Geometry: see drawing. Coordinates: mm, zero at the bounding-box minimum. A direction names the side the tool comes from. Give positions to 0.01 mm unless a question says otherwise; leave off trailing zeros. Loops run counter-clockwise (first coordinate to the right, second up) from the corner with the lowest first, then second, coordinate; pieces in that order, holes last. Notation, with made-up numbers: (7.5, 39) -> (36.5, 39) arc R23 ccw to (36.5, 48) -> close; hole circle Ø6 at (37, 70.5). An arc over 180 degrees is marked (long way). Return JSON: item names as keys, results as strings. Group by question number.
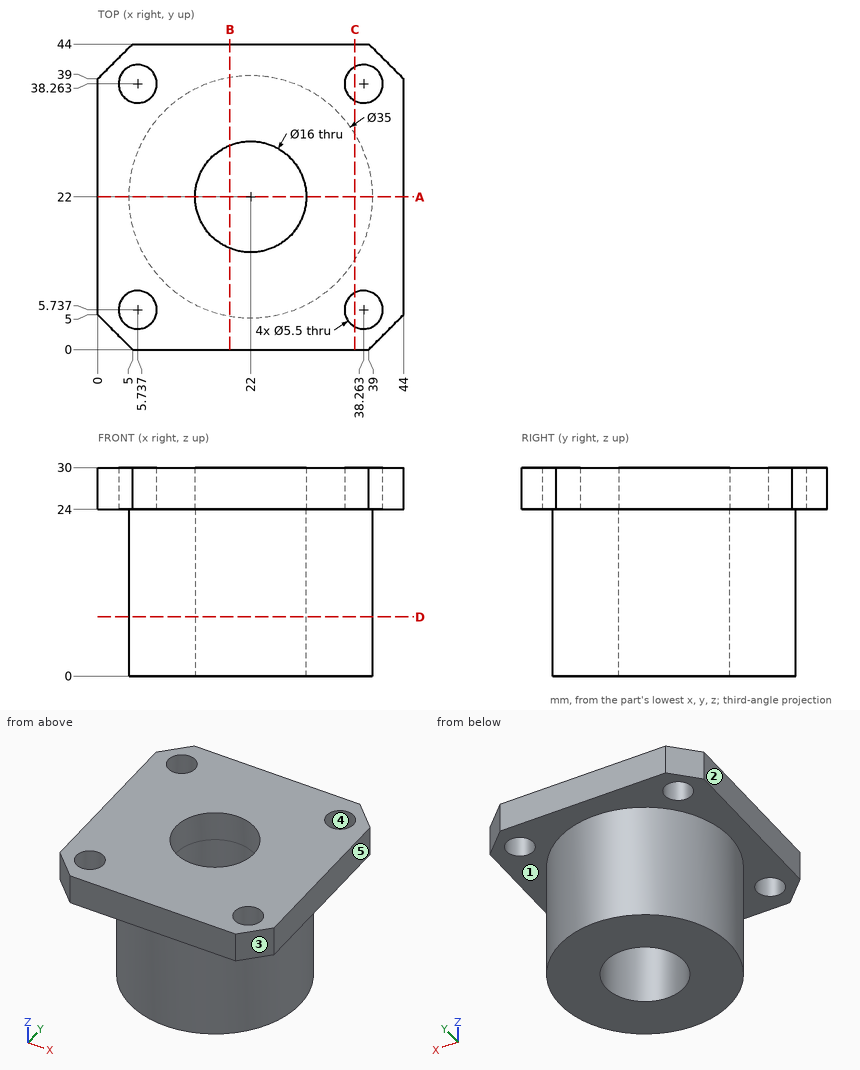
1) Mould query, pull axis Y, two halves, no side actions, for the marked faces 3, 4 and 5. Classes: released by +Y, released by -Y, zero draft, split by the parting line, or undercut.
2) Cut plane D-D on z = 8.5. Return loops of the section in (x, y), then the cut area to 3 significant figures.
3) Cut plane B-B on x = 19. Return loops of the section in (y, z).
4) Cut plane A-A on y = 22. Return loops of the section in (x, z), then the cut area to 3 significant figures.
5) Contact query for flat-ended pins moving along their axis: P1, Ø3, axis at x = 19.5, y = 7, coming from the -Z side; P2, Ø1.5, axis at y = 24, z = 19, coming from the -X side (1 decimal); P3, Ø7, axis at x = 5.74, y = 38.26, coming from the -Z side; P4, Ø4.5, axis at x = 5.74, y = 5.74, coming from the +Z side. Output: stop coordinate, or through.
6) Reachability of the marked faces 1 and 2 from +Z, -Z, +X, -X, +Y, -Y: full face, straight path, thin tool, end or side. Return the list, or none.
7) Cut plane C-C on x = 37. Return loops of the section in (y, z).
8) Material intervals for line 1 (Y direction, x = 22, z = 8.25); line 2 (Y direction, x = 22, z = 26); line 3 (Z direction, x = 37.5, y = 11.5), sorted ascending.
Calculated:
{
 "1": {"face 3": "released by -Y", "face 4": "undercut", "face 5": "zero draft"},
 "2": {"outline": "circle Ø35 at (22, 22); hole circle Ø16 at (22, 22)", "area": "761 mm2"},
 "3": {"outline": "(0, 24) -> (4.76, 24) -> (4.76, 0) -> (14.58, 0) -> (14.58, 30) -> (0, 30) -> close; (29.42, 0) -> (39.24, 0) -> (39.24, 24) -> (44, 24) -> (44, 30) -> (29.42, 30) -> close"},
 "4": {"outline": "(0, 24) -> (4.5, 24) -> (4.5, 0) -> (14, 0) -> (14, 30) -> (0, 30) -> close; (30, 0) -> (39.5, 0) -> (39.5, 24) -> (44, 24) -> (44, 30) -> (30, 30) -> close", "area": "624 mm2"},
 "5": {"P1": "z = 0", "P2": "x = 4.5", "P3": "z = 24", "P4": "through"},
 "6": {"face 1": "-Z", "face 2": "+Z, -Z, -X, +Y, -Y"},
 "7": {"outline": "(0, 24) -> (3.29, 24) -> (3.29, 30) -> (0, 30) -> close; (8.18, 24) -> (12.99, 24) -> (12.99, 0) -> (31.01, 0) -> (31.01, 24) -> (35.82, 24) -> (35.82, 30) -> (8.18, 30) -> close; (40.71, 24) -> (44, 24) -> (44, 30) -> (40.71, 30) -> close"},
 "8": {"line 1": "4.5 to 14, 30 to 39.5", "line 2": "0 to 14, 30 to 44", "line 3": "24 to 30"}
}
